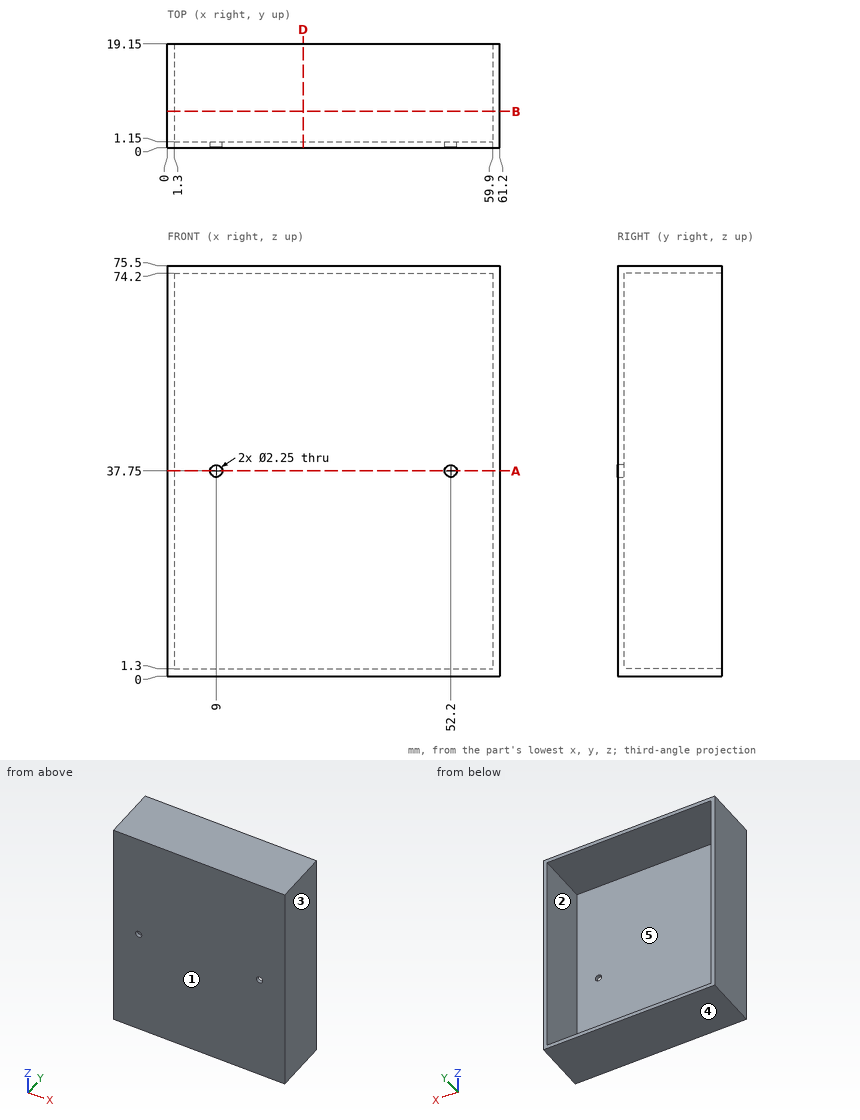
Study the drawing (mm; zero at the part's minimum x, y, z) and answer. A direction names the side the tool comes from. Round coordinates to 2 decimals unless told otherwise and drop trailing zeros. Write each loop counter-clockwise with the first axis right and the second up, starting at its lowest first coordinate (ties: lowest second). Pieces come first, ordered by that corner, then holes. Notation, with made-up numbers: (-31.75, 20.25) -> (12.25, 20.25) arc R24 cw to (12.25, 39.25) -> close; hole circle Ø5 at (17.5, 34.25). An arc over 180 degrees is marked (long way). Use CSV: the item, a comma, the result in double quotes. Start each with the question number.
(1) Each of these flat-tipped pins is pushed along its axis until it touches: pin 1 (1.8 mm diameter, centred on x = 52.2, z = 37.75, fed in from -Y); pin 2 (3.5 mm diameter, centred on x = 9, z = 37.75, fed in from +Y). Where does it stop, or does it pass through?
(2) Section B-B on y = 6.75 is taken. Give the vertices of the cut face in (x, z).
(3) Section D-D on x = 25 is taken. Give the vertices of the cut face in (y, z).
(4) Consider L1, parallel to X at y = 0.8, z = 37.75 (1 decimal); L2, parallel to X at y = 3.5, z = 51.5; L3, parallel to Z at x = 16, y = 12.75. Determine where each line is inside the solid, lowest interval first. Write a range as from..to.
(5) Section A-A on z = 37.75 is taken. Count the separate pieces of the cut face and the enclosed holes in it, then the cut area to 3 significant figures.
(6) The mould has two halves that part along X. Classify the marked faces 3, 4 and 5: released by +X, released by -X, zero draft, split by the parting line, or undercut.
(7) Which of the six approach directions +Z, -Z, +X, -X, +Y, -Y give full straight-line access (tool end or side, diameter ignored) to the marked faces 1 and 2?
A:
1,pin 1,"passes through"
1,pin 2,"stops at y = 1.15"
2,outline,"(0, 0) -> (61.2, 0) -> (61.2, 75.5) -> (0, 75.5) -> close; hole (1.3, 1.3) -> (59.9, 1.3) -> (59.9, 74.2) -> (1.3, 74.2) -> close"
3,outline,"(0, 0) -> (19.15, 0) -> (19.15, 1.3) -> (1.15, 1.3) -> (1.15, 74.2) -> (19.15, 74.2) -> (19.15, 75.5) -> (0, 75.5) -> close"
4,L1,"x = 0..7.9, 10.1..51.1, 53.3..61.2"
4,L2,"x = 0..1.3, 59.9..61.2"
4,L3,"z = 0..1.3, 74.2..75.5"
5,separate pieces,"3"
5,enclosed holes,"0"
5,area,"112 mm²"
6,face 3,"released by +X"
6,face 4,"zero draft"
6,face 5,"undercut"
7,face 1,"+Z, -Z, +X, -X, -Y"
7,face 2,"+Y"
